```python
from build123d import *

# Parameters (mm, degrees)
SKETCH7_R               = 1.5
CUT_EXTRUDE1_DEPTH      = 5
CHAMFER1_SIZE           = 0.2
SKETCH4_R               = 1.5
CUT_EXTRUDE2_DEPTH      = 13.5
CUT_EXTRUDE2_DEPTH_BACK = 13.5


with BuildPart() as part:
    # Sketch1 → Revolve1 (revolve)
    with BuildSketch(Plane(origin=(0, 0, 0), x_dir=(1, 0, 0), z_dir=(0, 1, 0))):
        Polygon((0, 0), (0, 32), (4, 32), (4, 12), (5, 12), (5, 4), (12.5, 4), (12.5, 0), align=None)
    revolve(axis=Axis((0, 0, 0), (0, 0, 1)))

    # Sketch7 → Cut-Extrude1 (cut, through all)
    with BuildSketch(Plane(origin=(0, 0, -4), x_dir=(-1, 0, 0), z_dir=(0, 0, -1))):
        with Locations((-9.5, 0)):
            Circle(SKETCH7_R)
        with Locations((0, 9.5)):
            Circle(SKETCH7_R)
        with Locations((9.5, 0)):
            Circle(SKETCH7_R)
        with Locations((0, -9.5)):
            Circle(SKETCH7_R)
    extrude(amount=-CUT_EXTRUDE1_DEPTH, mode=Mode.SUBTRACT)

    # Chamfer1
    chamfer1_edges = [part.edges().sort_by_distance(p)[0] for p in [
        (-5, 0, -12),
    ]]
    chamfer(chamfer1_edges, length=CHAMFER1_SIZE)

    # Sketch4 → Cut-Extrude2 (cut, two sides)
    with BuildSketch(Plane(origin=(0, 0, 0), x_dir=(1, 0, 0), z_dir=(0, 1, 0))) as cut_extrude2_sk:
        with Locations((0, 28)):
            Circle(SKETCH4_R)
    extrude(amount=CUT_EXTRUDE2_DEPTH, mode=Mode.SUBTRACT)
    extrude(cut_extrude2_sk.sketch, amount=-CUT_EXTRUDE2_DEPTH_BACK, mode=Mode.SUBTRACT)


solid = part.part
```
Build history of the part. All positions in model axes, mm. A direction names the side the tool comes from. Coordinates: 2 decimals unless noted, no trailing zeros. Order: outer loops, then holes, each group sorted by start corner. A loop starts at its lowest first (then second) coordinate and runs counter-clockwise, first axis right, second up. Notation, with made-up numbers: (-26, 65) -> (-1, 65) arc R28 cw to (-1, 85) -> close; hole circle Ø7 at (38, -4.75). An arc over 180 degrees is marked (long way). Answer in a Markdown table with one row per item. Add a question column.
Q1. Drop flat-ended pins along their axis: pin 1 (1.8 mm diameter, centred on x = -9.5, y = 0, fed in from +Z); pin 2 (5 mm diameter, centred on x = 0, y = -9.5, fed in from -Z); pin 3 (3 mm diameter, centred on y = 0, z = -22.5, fed in from -X); pin 4 (8 mm diameter, centred on y = -3, z = -13.5, fed in from +X). Give the stop position or say it passes through.
Q2. Band-saw the part on B-B, the plane x = 9.5. List the corners of the cut face in (y, z).
Q3. Which spindle directions (+Z, -Z, +X, -X, +Y, -Y) get a long thin tool onto all of the face, cutting with end or side? Do faces 4 (the face through (3.695, -1.532, -21.86)), 5 (the face through (-0.195, 0.056, -29.487)). Say none if no direction does.
Q4. Wall check: line 1 along Y through (x, z) = (0, -2.65); line 2 along Z through (x, y) = (-8.5, -9); line 3 along Y through (x, z) = (-9.5, -1.8). Give the ranges that are in metal, low to high. Write a range as [from, to].
Q5. Band-saw the part on C-C, the plane y = -10.25. List the corners of the cut face in (x, z), then the cut area to 3 significant figures.
Q6. Band-saw the part on A-A, the plane y = 0. List the corners of the cut face in (x, z), then the cut area to 3 significant figures.
Q7. Mould opens along X. For faces 1 (the face through (0, -11, -2)), 2 (the face through (11.923, 3.755, -1.972)), 3 (the face through (0, 0, -32)) say: +X half, -X half, draft (parallel to the pull), parting line (faces both ways), or undercut.
Q8. Band-saw the part on D-D, the plane z = -14. List the corners of the cut face in (x, y).
Answers follow:
| question | item | result |
|---|---|---|
| 1 | pin 1 | through |
| 1 | pin 2 | z = -4 |
| 1 | pin 3 | x = -4 |
| 1 | pin 4 | x = 5 |
| 2 | outline | (-8.12, -4) -> (-1.5, -4) -> (-1.5, 0) -> (-8.12, 0) -> close; (1.5, -4) -> (8.12, -4) -> (8.12, 0) -> (1.5, 0) -> close |
| 3 | face 4 | -Z |
| 3 | face 5 | +Y, -Y |
| 4 | line 1 | [-12.5, -11], [-8, 8], [11, 12.5] |
| 4 | line 2 | [-4, 0] |
| 4 | line 3 | [-8.12, -1.5], [1.5, 8.12] |
| 5 | outline | (-7.15, -4) -> (-1.3, -4) -> (-1.3, 0) -> (-7.15, 0) -> close; (1.3, -4) -> (7.15, -4) -> (7.15, 0) -> (1.3, 0) -> close |
| 5 | area | 46.8 mm^2 |
| 6 | outline | (-12.5, -4) -> (-11, -4) -> (-11, 0) -> (-12.5, 0) -> close; (-8, -4) -> (-5, -4) -> (-5, -11.8) -> (-4.8, -12) -> (-4, -12) -> (-4, -32) -> (4, -32) -> (4, -12) -> (4.8, -12) -> (5, -11.8) -> (5, -4) -> (8, -4) -> (8, 0) -> (-8, 0) -> close; (11, -4) -> (12.5, -4) -> (12.5, 0) -> (11, 0) -> close; hole circle Ø3 at (0, -28) |
| 6 | area | 309 mm^2 |
| 7 | face 1 | undercut |
| 7 | face 2 | parting line |
| 7 | face 3 | draft |
| 8 | outline | circle Ø8 at (0, 0) |
